Geometry: see drawing. Coordinates: mm, zero at the bounding-box minimum. Coordinates: 2 decimals unless noted, no trailing zeros. Write each loop counter-clockwise with the first axis right and the second up, starting at its lowest first coordinate (ties: lowest second). Pieces come first, ordered by that corner, then holes. Notation, with made-up numbers: (-13, 14.25) - (20, 14.25) arc R24 ccw to (20, 46.25) - close; hole circle Ø9 at (40, 88.25). An arc over 180 degrees is marked (long way). One line per question, with ' | ' between items. Start each with the question number.
Q1. Contact query for a flat-ended pin moving along its axis: P1, Ø6, axis at x = 56, z = 752, coming from the +Y side. Output: stop coordinate, or through.
Q2. Line query: line 1 (X direction, y = 35.5, z = 752); line 2 (Z direction, x = 56, y = 23); line 3 (Z direction, x = 56, y = 15). Output: solid intervals per line, ascending.
Q3. Cut plane A-A, the plane x = 35. Return loops of the section in (y, z).
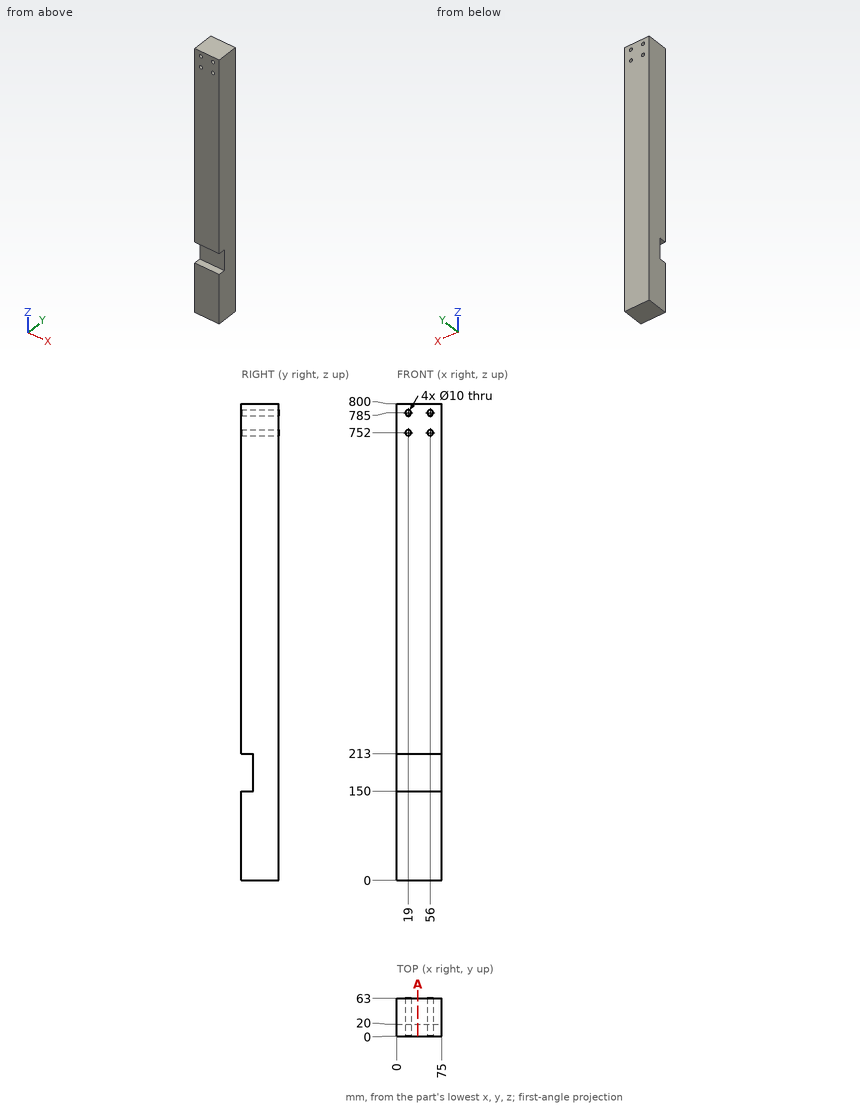
Reply:
1) P1: passes through
2) line 1: x = 0 to 14, 24 to 51, 61 to 75 | line 2: z = 0 to 747, 757 to 780, 790 to 800 | line 3: z = 0 to 150, 213 to 747, 757 to 780, 790 to 800
3) outline: (0, 0) - (63, 0) - (63, 800) - (0, 800) - (0, 213) - (20, 213) - (20, 150) - (0, 150) - close
